Check sheet for the modelled part. Datum: model origin and axes. Units: mm. Face numbers are marked on the shaded views. A direction names the side the tool comes from. Round coordinates to 2 decimals unless told otherwise and drop trailing zeros. Write each loop counter-clockwise with the first axis right and the second up, starting at its lowest first coordinate (ties: lowest second). Pieces come first, ordered by that corner, then holes. Notation, with made-up numbers: (-39.75, 30) -> (-4.75, 30) arc R29 cw to (-4.75, 54) -> close; hole circle Ø9 at (87.25, 33.25). An arc over 180 degrees is marked (long way). One line per item, written item: value.
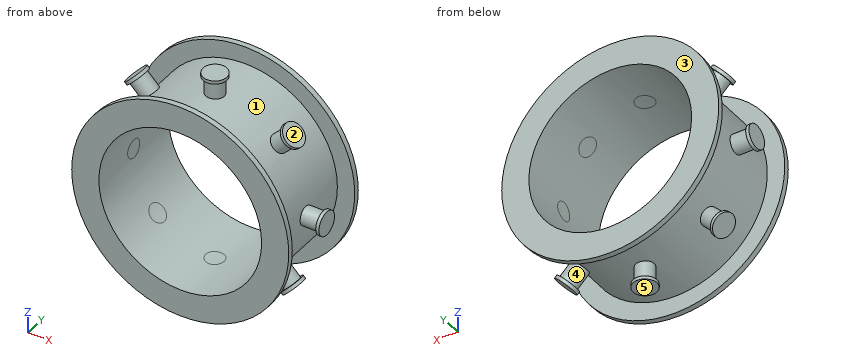
from build123d import *

# Parameters (mm, degrees)
F0_R            = 12.7
F0_R_2          = 9.525
F1_DEPTH        = 6.223
F2_R            = 15.24
F2_R_2          = 10.668
F3_DEPTH        = 5.588
F4_R            = 1.0795
F6_DEPTH        = 12.7
F6_COPIES_COUNT = 8
F7_R            = 1.397
F8_DEPTH        = 0.381
F8_COPIES_COUNT = 8
F9_R            = 9.525
F10_DEPTH       = 12.4470001


# Not quite as in the source:
# - a pattern or mirror of a feature is missing from the dataset's text; its kind, count and spacing are read off the source's solid


with BuildPart() as f1:
    # F0 (on Front) → F1 (new body, symmetric)
    with BuildSketch(Plane.XZ):
        Circle(F0_R)
        Circle(F0_R_2, mode=Mode.SUBTRACT)
    extrude(amount=F1_DEPTH, both=True)

    # F2 (on Front) → F3 (cut, symmetric)
    with BuildSketch(Plane.XZ):
        Circle(F2_R)
        Circle(F2_R_2, mode=Mode.SUBTRACT)
    extrude(amount=F3_DEPTH, both=True, mode=Mode.SUBTRACT)

    # F4 (on Right) → F6 (join)
    with BuildSketch(Plane.YZ):
        Circle(F4_R)
    f6 = extrude(amount=-F6_DEPTH)

    # F6_copies: F6 ×8 about axis
    f6_copies_axis = Axis((0, 0, 0), (0, 1, 0))
    for i in range(1, F6_COPIES_COUNT):
        add(f6.rotate(f6_copies_axis, i * 360 / F6_COPIES_COUNT))

    # F7 (on face) → F8 (join)
    with BuildSketch(Plane(origin=(-12.7, 0, 0), x_dir=(0, -1, 0), z_dir=(-1, 0, 0))):
        Circle(F7_R)
    f8 = extrude(amount=F8_DEPTH)

    # F8_copies: F8 ×8 about axis
    f8_copies_axis = Axis((0, 0, 0), (0, 1, 0))
    for i in range(1, F8_COPIES_COUNT):
        add(f8.rotate(f8_copies_axis, i * 360 / F8_COPIES_COUNT))

    # F9 (on face) → F10 (cut, through all)
    with BuildSketch(Plane.XZ.offset(6.223)):
        Circle(F9_R)
    extrude(amount=-F10_DEPTH, mode=Mode.SUBTRACT)


solid = f1.part
Item 1: Sectioned sample at C-C on y = -4. Enter the section's corners in (x, z) (3 decimals), and give its area (3 significant figures).
Answer:
outline: circle Ø21.336 at (0, 0); hole circle Ø19.05 at (0, 0)
area: 72.5 mm^2
Item 2: Thickness scan on line 1 (Z direction, x = 0, y = 3.75) (3 decimals); line 2 (Z direction, x = 0, y = 1) (3 decimals). Record the ranges inside material, lowest first.
Answer:
line 1: z = -10.668 to -9.525, 9.525 to 10.668
line 2: z = -13.081 to -9.525, 9.525 to 13.081
Item 3: Depth check by flat-ended pin: P1, Ø1.5, axis at x = -8.5, y = 1.5, coming from the +Z side; P2, Ø1, axis at x = -9.5, y = -2, coming from the +Z side; P3, Ø1.5, axis at x = -6.5, z = 6.5, coming from the +Y side; P4, Ø1, axis at y = 5, z = 5, coming from the +X side. Enter the tip coordinate at first touch or a pass-through.
Answer:
P1: stops at z = 10.08
P2: stops at z = 5.73
P3: stops at y = 6.22
P4: stops at x = 9.67
Item 4: Tool access check on the marked faces 1 and 2. Record the directions out of +Z, -Z, +X, -X, +Y, -Y that give a thin tool (end or side, any length) a straight path to the whole face; none if there is none.
Answer:
face 1: none
face 2: +Z, +X, +Y, -Y
Item 5: Sectioned sample at D-D on x = -5. Enter the section's corners in (y, z).
Answer:
outline: (-6.22, -11.67) -> (-5.59, -11.67) -> (-5.59, -9.42) -> (5.59, -9.42) -> (5.59, -11.67) -> (6.22, -11.67) -> (6.22, -8.11) -> (-6.22, -8.11) -> close; (-6.22, 8.11) -> (6.22, 8.11) -> (6.22, 11.67) -> (5.59, 11.67) -> (5.59, 9.42) -> (-5.59, 9.42) -> (-5.59, 11.67) -> (-6.22, 11.67) -> close
Item 6: Mould release check, pull along Z, two halves, no side actions. Record for the marked faces 3, 4 and 5: pulls with the +Z half, pulls with the -Z half, needs draft (parallel to the pull), parting line crosses it, or undercut.
Answer:
face 3: needs draft
face 4: undercut
face 5: pulls with the -Z half
